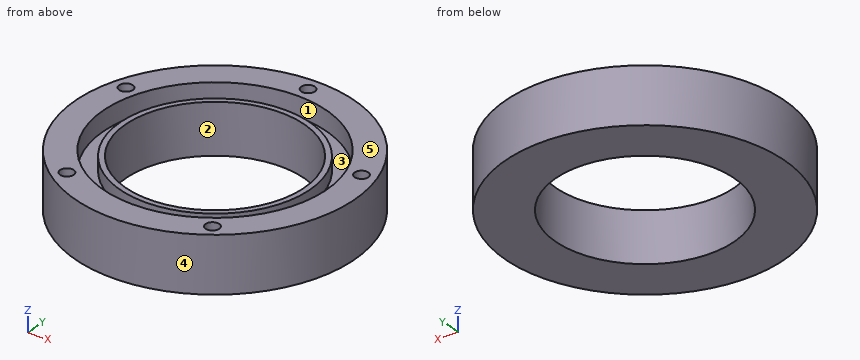
Autodesk Inventor part; units mm, degrees
ref_plane "YZ Plane" through (0, 0, 0) normal (1, 0, 0) x (0, 1, 0)
ref_plane "XZ Plane" through (0, 0, 0) normal (0, 1, 0) x (-1, 0, 0)
ref_plane "XY Plane" through (0, 0, 0) normal (0, 0, 1) x (1, 0, 0)
sketch "Sketch2" plane through (0, 0, 0) normal (0, 0, 1) x (1, 0, 0)
  circle A0 centre (0, 0) radius 25
  circle A1 centre (0, 0) radius 16
  dimension "d0" = 50
  dimension "d1" = 32
extrude "Extrusion1" add sketch "Sketch2" along normal blind 10
sketch "Sketch3" plane through (0, 0, 10) normal (0, 0, 1) x (1, 0, 0)
  circle A0 centre (0, 0) radius 25 construction
  circle A1 centre (0, 0) radius 16 construction
  circle A2 centre (0, 0) radius 16
  circle A3 centre (0, 0) radius 20
  dimension "d4" = 4
extrude "Extrusion2" cut sketch "Sketch3" against normal blind 1
sketch "Sketch4" plane through (0, 0, 9) normal (0, 0, 1) x (1, 0, 0)
  circle A0 centre (0, 0) radius 20 construction
  circle A1 centre (0, 0) radius 16 construction
  circle A2 centre (0, 0) radius 20
  circle A3 centre (0, 0) radius 17
  dimension "d7" = 1
  dimension "d8" = 40
  dimension "d9" = 34
extrude "Extrusion3" cut sketch "Sketch4" against normal blind 2.5
sketch "Sketch5" plane through (0, 0, 10) normal (0, 0, 1) x (1, 0, 0)
  line L0 (0, 35) -> (0, -35) construction
  circle A0 centre (0, 0) radius 20 construction
  point P0 (0, 22.5)
  point P1 (-21.3988, 6.9529)
  point P2 (-13.2252, -18.2029)
  point P3 (13.2252, -18.2029)
  point P4 (21.3988, 6.9529)
  dimension "d12" = 22.5
  dimension "d15" = 360
hole "Hole1" at (-21.3988, 6.9529, 10) at (0, 22.5, 10) at (21.3988, 6.9529, 10) at (13.2252, -18.2029, 10) at (-13.2252, -18.2029, 10) direction (0, 0, -1) diameter 2.459 depth 8.8 tip angle 118
properties part number "P029_BasEcranProtecCam"
Build history of the part. All positions in model axes, mm. Face numbers are marked on the shaded views. A direction names the side the tool comes from. Round coordinates to 2 decimals unless told otherwise and drop trailing zeros. Write each loop counter-clockwise with the first axis right and the second up, starting at its lowest first coordinate (ties: lowest second). Pieces come first, ordered by that corner, then holes. Notation, with made-up numbers: (14.25, 84.5) -> (45.25, 84.5) arc R25 ccw to (45.25, 102.5) -> close; hole circle Ø9 at (-34, 33.25). An arc over 180 degrees is marked (long way). Write item = value, one per line.
(1) Probe L1, parallel to Y at x = 0, z = 8; L2, parallel to X at y = 0.5, z = 7 (3 decimals); L3, parallel to X at y = 7, z = 1.25. List the from-to ranges inside material, lowest first.
Answer:
L1 = -25 to -20, -17 to -16, 16 to 17, 20 to 21.27, 23.73 to 25
L2 = -24.995 to -19.994, -16.993 to -15.992, 15.992 to 16.993, 19.994 to 24.995
L3 = -24 to -22.63, -20.17 to -14.39, 14.39 to 20.17, 22.63 to 24
(2) Band-saw the part on A-A (y = 0). Give the cut face in (x, z), then the cut area to 3 significant figures.
Answer:
outline = (-25, 0) -> (-16, 0) -> (-16, 9) -> (-17, 9) -> (-17, 6.5) -> (-20, 6.5) -> (-20, 10) -> (-25, 10) -> close; (16, 0) -> (25, 0) -> (25, 10) -> (20, 10) -> (20, 6.5) -> (17, 6.5) -> (17, 9) -> (16, 9) -> close
area = 157 mm2
(3) Band-saw the part on B-B (x = -6). Give the cut face in (y, z).
Answer:
outline = (-24.27, 0) -> (-14.83, 0) -> (-14.83, 9) -> (-15.91, 9) -> (-15.91, 6.5) -> (-19.08, 6.5) -> (-19.08, 10) -> (-24.27, 10) -> close; (14.83, 0) -> (24.27, 0) -> (24.27, 10) -> (19.08, 10) -> (19.08, 6.5) -> (15.91, 6.5) -> (15.91, 9) -> (14.83, 9) -> close
(4) Tool access for the marked faces 1 and 2: list every direction of +Z, -Z, +X, -X, +Y, -Y with a clear straight run to the whole face (end or side of a thin tool).
Answer:
face_1 = +Z
face_2 = +Z, -Z
(5) Two-plate mould, pull along X, no slides. Class the marked faces 3, 4 and 5: pulls with the +X half, pulls with the -X half, needs draft (parallel to the pull), parting line crosses it, or undercut.
Answer:
face_3 = undercut
face_4 = parting line crosses it
face_5 = needs draft
(6) Flat gauge pins, fed straight in: pin 1 (4 mm diameter, centred on y = 14.5, z = 8.5, fed in from -X); pin 2 (2 mm diameter, centred on x = 0, y = 22.5, fed in from +Z); pin 3 (12 mm diameter, centred on x = 1.5, y = 4, fed in from +Z); pin 4 (2 mm diameter, centred on x = 10, z = 2.5, fed in from -Y). Where does each tip first touch, or does it go through?
Answer:
pin_1 = -21.65
pin_2 = 1.06
pin_3 = through
pin_4 = -23.32
